Could you check a few things on this model? Use its own coordinates, in mm. Face numbers are marked on the shaded views. A direction names the side the tool comes from. Give positions to 0.01 mm unless a question says otherwise; leave off trailing zeros. Loops run counter-clockwise (first coordinate to the right, second up) from the corner with the lowest first, then second, coordinate; pieces in that order, holes last. Notation, with made-up numbers: M 51,61.25 L 88,61.25 A26 ccw 88,88.25 Z; hole C 62,-12.75 d7. An arc over 180 degrees is marked long. Return JSON: item names as keys, results as strings. Group by question number.
1. For the marked faces 1, 2 and 3, which set-ups out of +Z, -Z, +X, -X, +Y, -Y let a thin tool reach every point of the face, with its end or its side?
2. If we section it at A-A (x = -114.3): Write out the boundary of the cut face in (y, z) (3 decimals), plus the area to 3 significant figures.
3. If we section it at B-B (z = 0): Write out the boundary of the cut face in (x, y) (3 decimals), plus the area to 3 significant figures.
4. If we mould it in two halves opening along Z, with no side actions, what happens to the marked faces 4, 5 and 6? For each: +Z half, -Z half, draft (parallel to the pull), parting line (faces both ways), or undercut.
5. For pin 1 (10 mm diameter, centred on x = -34, z = -6.5, fed in from +Y); pin 2 (5 mm diameter, centred on y = 5, z = 9.5, fed in from -X); pin 3 (7.5 mm diameter, centred on x = -66.5, z = -1, fed in from -Y), each with a flat end and sliding along its axis, tell me the tip position at first contact or that it passes through.
6. If we section it at D-D (x = 88.9): Write out the boundary of the cut face in (y, z).
7. If we section it at C-C (y = 2): Write out the boundary of the cut face in (x, z) (3 decimals).
8. Please list where these lines run through material, in increasing order: line 1 (X direction, y = 0, z = -0.5); line 2 (Z direction, x = -114, y = 0); line 3 (X direction, y = -15, z = -0.25).
```python
from build123d import *

# Parameters (mm, degrees)
F0_R     = 9.525
F1_DEPTH = 6.35
F2_R     = 6.35
F3_DEPTH = 12.7
F4_R     = 6.35
F5_DEPTH = 12.7


with BuildPart() as f1:
    # F0 (on Front) → F1 (new body, symmetric)
    with BuildSketch(Plane.XZ):
        with BuildLine():
            ThreePointArc((101.6, 6.35), (99.740128, 10.840128), (95.25, 12.7))
            Line((95.25, 12.7), (-120.65, 12.7))
            ThreePointArc((-120.65, 12.7), (-125.140128, 10.840128), (-127, 6.35))
            Line((-127, 6.35), (-127, -6.35))
            ThreePointArc((-127, -6.35), (-125.140128, -10.840128), (-120.65, -12.7))
            Line((-120.65, -12.7), (95.25, -12.7))
            ThreePointArc((95.25, -12.7), (99.740128, -10.840128), (101.6, -6.35))
            Line((101.6, -6.35), (101.6, 6.35))
        make_face()
        with Locations((-114.3, 0)):
            Circle(F0_R, mode=Mode.SUBTRACT)
    extrude(amount=F1_DEPTH, both=True)

    # F2 (on face) → F3 (join)
    with BuildSketch(Plane.XZ.offset(6.35)):
        with Locations((88.9, 0)):
            Circle(F2_R)
    extrude(amount=F3_DEPTH)

    # F4 (on face) → F5 (join)
    with BuildSketch(Plane(origin=(0, 6.35, 0), x_dir=(-1, 0, 0), z_dir=(0, 1, 0))):
        Circle(F4_R)
    extrude(amount=F5_DEPTH)


solid = f1.part
```
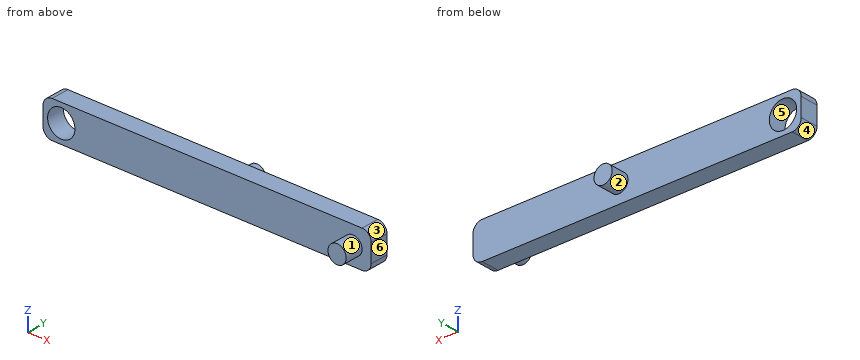
Answer:
{
 "1": {"face 1": "-Y", "face 2": "+Y", "face 3": "+Z, +X, +Y, -Y"},
 "2": {"outline": "M -6.35,-12.7 L 6.35,-12.7 L 6.35,-9.525 L -6.35,-9.525 Z; M -6.35,9.525 L 6.35,9.525 L 6.35,12.7 L -6.35,12.7 Z", "area": "80.6 mm²"},
 "3": {"outline": "M -127,-6.35 L -123.825,-6.35 L -123.825,6.35 L -127,6.35 Z; M -104.775,-6.35 L 82.55,-6.35 L 82.55,-19.05 L 95.25,-19.05 L 95.25,-6.35 L 101.6,-6.35 L 101.6,6.35 L 6.35,6.35 L 6.35,19.05 L -6.35,19.05 L -6.35,6.35 L -104.775,6.35 Z", "area": "2,980 mm²"},
 "4": {"face 4": "-Z half", "face 5": "undercut", "face 6": "draft"},
 "5": {"pin 1": "stops at y = 6.35", "pin 2": "stops at x = -126.97", "pin 3": "stops at y = -6.35"},
 "6": {"outline": "M -19.05,-6.35 L -6.35,-6.35 L -6.35,-12.7 L 6.35,-12.7 L 6.35,12.7 L -6.35,12.7 L -6.35,6.35 L -19.05,6.35 Z"},
 "7": {"outline": "M -127,-6.35 A6.35 ccw -120.65,-12.7 L 95.25,-12.7 A6.35 ccw 101.6,-6.35 L 101.6,6.35 A6.35 ccw 95.25,12.7 L -120.65,12.7 A6.35 ccw -127,6.35 Z; hole C -114.3,0 d19.05"},
 "8": {"line 1": "x = -127 to -123.81, -104.79 to 101.6", "line 2": "z = -12.7 to -9.52, 9.52 to 12.7", "line 3": "x = 82.55 to 95.25"}
}
